Build history of the part. All positions in model axes, mm. A direction names the side the tool comes from. Round coordinates to 2 decimals unless told otherwise and drop trailing zeros. Write each loop counter-clockwise with the first axis right and the second up, starting at its lowest first coordinate (ties: lowest second). Pieces come first, ordered by that corner, then holes. Notation, with made-up numbers: (30.25, -38.75) - (34.25, -38.75) arc R8 cw to (34.25, -27.75) - close; hole circle Ø10 at (21.5, -21.75). An arc over 180 degrees is marked (long way). One line per question, with ' | ' between items.
from build123d import *

# Parameters (mm, degrees)
SKETCH3_W                              = 178.001
SKETCH3_H                              = 211.818599984
BOSS_EXTRUDE1_DEPTH                    = 8.466666582
F_18_0_1695_DIAMETER_HOLE1_D           = 4.3053
F_18_0_1695_DIAMETER_HOLE1_CSINK_D     = 5.5753
F_18_0_1695_DIAMETER_HOLE1_CSINK_ANGLE = 90
CUT_EXTRUDE1_DEPTH                     = 5.08
CUT_EXTRUDE2_DEPTH                     = 5.08
CHAMFER1_SIZE                          = 0.635


with BuildPart() as part:
    # Sketch3 → Boss-Extrude1 (new body)
    with BuildSketch(Plane.XY):
        with Locations((2.3495, -14.559299992)):
            Rectangle(SKETCH3_W, SKETCH3_H)
        Polygon((-33.01966, 85), (73.75034, 85), (73.75034, -114.118599984), (-68.48966, -114.118599984), (-68.48966, 72.39), (-45.62966, 72.39), align=None, mode=Mode.SUBTRACT)
    extrude(amount=-BOSS_EXTRUDE1_DEPTH)

    # #18 (0.1695) Diameter Hole1 (through all)
    with Locations(Plane(origin=(0, 0, 0), x_dir=(-1, 0, 0), z_dir=(0, 0, 1))):
        with Locations((51.97966, -78.74), (74.83966, 78.74), (-80.10034, 78.74), (-80.10034, -78.74)):
            CounterSinkHole(F_18_0_1695_DIAMETER_HOLE1_D / 2, F_18_0_1695_DIAMETER_HOLE1_CSINK_D / 2, counter_sink_angle=F_18_0_1695_DIAMETER_HOLE1_CSINK_ANGLE)

    # Sketch9 → Cut-Extrude1 (cut)
    with BuildSketch(Plane.ZY.offset(86.651)):
        Polygon((-4.233333333, -65.0886), (-1.058333333, -68.2636), (-4.233333333, -71.4386), (-7.408333333, -68.2636), align=None)
        Polygon((-4.233333333, 90.291666667), (-1.058333333, 87.116666667), (-4.233333333, 83.941666667), (-7.408333333, 87.116666667), align=None)
    extrude(amount=-CUT_EXTRUDE1_DEPTH, mode=Mode.SUBTRACT)

    # Sketch10 → Cut-Extrude2 (cut)
    with BuildSketch(Plane.XZ.offset(120.468599984)):
        Polygon((-85.592666667, -4.233333333), (-82.417666667, -1.058333333), (-79.242666667, -4.233333333), (-82.417666667, -7.408333333), align=None)
        Polygon((83.941666667, -4.233333333), (87.116666667, -1.058333333), (90.291666667, -4.233333333), (87.116666667, -7.408333333), align=None)
    extrude(amount=-CUT_EXTRUDE2_DEPTH, mode=Mode.SUBTRACT)

    # Chamfer1
    chamfer1_edges = [part.edges().sort_by_distance(p)[0] for p in [
        (88.704166667, -115.388599984, -2.645833333),
        (88.704166667, -115.388599984, -5.820833333),
        (85.529166667, -120.468599984, -5.820833333),
        (88.704166667, -120.468599984, -5.820833333),
        (88.704166667, -120.468599984, -2.645833333),
        (85.529166667, -120.468599984, -2.645833333),
        (-81.571, -66.6761, -5.820833333),
        (-81.571, -66.6761, -2.645833333),
        (-81.571, -69.8511, -2.645833333),
        (-81.571, -69.8511, -5.820833333),
        (-86.651, -66.6761, -5.820833333),
        (-86.651, -69.8511, -5.820833333),
        (-86.651, -69.8511, -2.645833333),
        (-86.651, -66.6761, -2.645833333),
        (-81.571, 88.704166667, -5.820833333),
        (-81.571, 88.704166667, -2.645833333),
        (-81.571, 85.529166667, -2.645833333),
        (-81.571, 85.529166667, -5.820833333),
        (-86.651, 88.704166667, -5.820833333),
        (-86.651, 85.529166667, -5.820833333),
        (-86.651, 85.529166667, -2.645833333),
        (-86.651, 88.704166667, -2.645833333),
        (-84.005166667, -115.388599984, -5.820833333),
        (-84.005166667, -115.388599984, -2.645833333),
        (-80.830166667, -115.388599984, -2.645833333),
        (-80.830166667, -115.388599984, -5.820833333),
        (-84.005166667, -120.468599984, -5.820833333),
        (-80.830166667, -120.468599984, -5.820833333),
        (-80.830166667, -120.468599984, -2.645833333),
        (-84.005166667, -120.468599984, -2.645833333),
        (85.529166667, -115.388599984, -5.820833333),
        (85.529166667, -115.388599984, -2.645833333),
    ]]
    chamfer(chamfer1_edges, length=CHAMFER1_SIZE)


solid = part.part
Q1. Saw through at A-A, the plane y = -8. List the corners of the cut face in (x, z).
Found:
outline: (-86.65, -8.47) - (-68.49, -8.47) - (-68.49, 0) - (-86.65, 0) - close; (73.75, -8.47) - (91.35, -8.47) - (91.35, 0) - (73.75, 0) - close
Q2. Drop flat-ended pins along their axis: pin 1 (4 mm diameter, centred on x = -51.98, y = 78.74, fed in from +Z); pin 2 (3.5 mm diameter, centred on x = 87, z = -5, fed in from -Y); pin 3 (5 mm diameter, centred on x = 80.1, y = -78.74, fed in from -Z); pin 4 (3.5 mm diameter, centred on y = -69.5, z = -4, fed in from -X). Give the stop position or say it passes through.
Found:
pin 1: through | pin 2: y = -119.96 | pin 3: z = -8.47 | pin 4: x = -86.56
Q3. Saw through at B-B, the plane x = -59. List the corners of the cut face in (y, z).
Found:
outline: (-120.47, -8.47) - (-114.12, -8.47) - (-114.12, 0) - (-120.47, 0) - close; (72.39, -8.47) - (91.35, -8.47) - (91.35, 0) - (72.39, 0) - close
Q4. Drill centre lines: L1, parallel to X at y = -78.74, z = -2; L2, parallel to X at y = 45, z = -4.5; L3, parallel to Y at x = -65.5, z = -6.25. Where is each one in solid material? Low to high. Write a range as from..to.
Found:
L1: -86.65..-76.99, -72.69..-68.49, 73.75..77.95, 82.25..91.35 | L2: -86.65..-68.49, 73.75..91.35 | L3: -120.47..-114.12, 72.39..91.35
Q5. Pull direction Y, two halves, no side cores. Call faces 1 (the flat face through (-71, -22, -8.467)), 2 (the flat face through (1, -120.469, -4)), 3 (the cylindrical face through (-72.786, -79.387, -4.606)): +Y half, -Y half, draft (parallel to the pull), parting line (faces both ways), or undercut.
Found:
face 1: draft | face 2: -Y half | face 3: undercut
Q6. Which spindle directions (+Z, -Z, +X, -X, +Y, -Y) get a long thin tool onto all of the face, cutting with end or side? Do faces 4 (the flat face through (-82, -115.389, -4)), 5 (the flat face through (-81.571, 87, -4)), 6 (the flat face through (-68.49, -22, -4)). Say none if no direction does.
Found:
face 4: -Y | face 5: -X | face 6: +Z, -Z
